The model under review builds one solid part; all positions refer to its coordinate system, in mm. Face numbers are marked on the shaded views. A direction names the side the tool comes from. Round coordinates to 2 decimals unless told otherwise and drop trailing zeros. Order: outer loops, then holes, each group sorted by start corner. A loop starts at its lowest first (then second) coordinate and runs counter-clockwise, first axis right, second up. Notation, with made-up numbers: M -18,22.25 L 23,22.25 A11 cw 23,30.25 Z; hole C -4,53.5 d10. An arc over 180 degrees is marked long. Answer as a JSON object with one key per item and string values. Group by question number.
1) Consider section A-A, the plane y = 0. Write out the cut boundary in (x, z), then the cut area to 4 significant figures.
2) Insertion check: pin 1 Ø1 at (x, z) = (-3, 2) entering from +Y; pin 2 Ø4 at (x, y) = (-3, 3.5) entering from +Z; pin 3 Ø2 at (x, y) = (1, 5) entering from +Z; pin 4 Ø1.5 at (y, z) = (0, 15.5) entering from +X. Each pin has a flat end and moves straight along its axis. Give the tip position at first contact, or say it passes through.
3) The part is to be moulded in two halves that separate along X. For the marked faces 1, 2 and 3, say which applies: +X half, -X half, draft (parallel to the pull), parting line (faces both ways), or undercut.
4) Consider section B-B, the plane z = 7.5. Write out the cut boundary in (x, y).
5) Consider section C-C, the plane z = 12. Write out the cut boundary in (x, y).
6) Consider section D-D, the plane y = -6.5. Write out the cut boundary in (x, z).
7) For the marked faces 4, 5 and 6, list the 3-axis set-ups (+Z, -Z, +X, -X, +Y, -Y) from which the entire face can be reached by the end or side of a thin tool; tool diameter is ignored.
8) To check wall thickness, follow line 1 (Z direction, x = 3.5, y = 4); line 2 (Y direction, x = -0.75, z = 18.25); line 3 (Y direction, x = -1.25, z = 19.25). State the ranges of each line that lie inside material, in increasing order.
```python
from build123d import *

# Parameters (mm, degrees)
PAD_DEPTH = 5


with BuildPart() as part:
    # Sketch → Revolution (revolve)
    with BuildSketch(Plane.XZ):
        Polygon((0, 20), (0, 0), (1.5, 0), (5, 3), (5, 10), (3, 10), (3, 20), align=None)
    revolve(axis=Axis((0, 0, 0), (0, 0, 1)))

    # Sketch001 (on Face4 of Revolution) → Pad (new body)
    with BuildSketch(Plane(origin=(0, 0, 10), x_dir=(-1, 0, 0), z_dir=(0, 0, 1))):
        Polygon((6.5, 3.752777), (0, 7.505553), (-6.5, 3.752777), (-6.5, -3.752777), (0, -7.505553), (6.5, -3.752777), align=None)
    extrude(amount=-PAD_DEPTH)

    # Sketch002 → Groove (revolve, cut)
    with BuildSketch(Plane.XZ):
        Polygon((1.75, 20), (0, 20), (0, 0), (1, 0), align=None)
    revolve(axis=Axis((0, 0, 0), (0, 0, 1)), mode=Mode.SUBTRACT)


solid = part.part
```
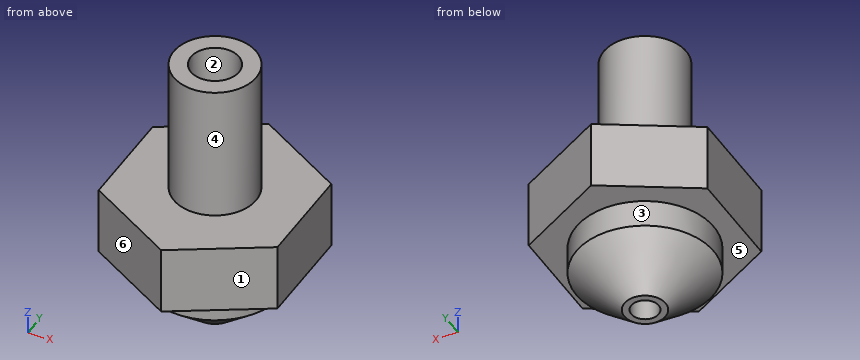
Results list:
{
 "1": {"outline": "M -6.5,5 L -5,5 L -5,3 L -1.5,0 L -1,0 L -1.75,20 L -3,20 L -3,10 L -6.5,10 Z; M 1,0 L 1.5,0 L 5,3 L 5,5 L 6.5,5 L 6.5,10 L 3,10 L 3,20 L 1.75,20 Z", "area": "109.5 mm^2"},
 "2": {"pin 1": "y = 3.36", "pin 2": "z = 20", "pin 3": "z = 10", "pin 4": "x = 3"},
 "3": {"face 1": "+X half", "face 2": "undercut", "face 3": "parting line"},
 "4": {"outline": "M -6.5,-3.75 L 0,-7.51 L 6.5,-3.75 L 6.5,3.75 L 0,7.51 L -6.5,3.75 Z; hole C 0,0 d2.56"},
 "5": {"outline": "C 0,0 d6; hole C 0,0 d2.9"},
 "6": {"outline": "M -1.74,5 L 1.74,5 L 1.74,10 L -1.74,10 Z"},
 "7": {"face 4": "+Z", "face 5": "-Z", "face 6": "+Z, -Z, -X, -Y"},
 "8": {"line 1": "5 to 10", "line 2": "-2.9 to -1.51, 1.51 to 2.9", "line 3": "-2.73 to -1.18, 1.18 to 2.73"}
}
